Geometry: final body of the model. Coordinates: model frame, mm. A direction names the side the tool comes from. Coordinates: 2 decimals unless noted, no trailing zeros. Loops run counter-clockwise (first coordinate to the right, second up) from the corner with the lowest first, then second, coordinate; pieces in that order, holes last. Notation, with made-up numbers: (5, 35.25) -> (34, 35.25) arc R22 ccw to (34, 47.25) -> close; hole circle Ø6 at (33.5, -3.5). An arc over 180 degrees is marked (long way). One line per item, written item: value. Start each with the question number.
Item 1: Set-up query: faces 4 (the flat face through (-6, 0, -9)), 5 (the flat face through (-4.039, 1, -6)). Return all of +Z, -Z, +X, -X, +Y, -Y with unobstructed straight access to the full face (end or side cutting, diameter ignored); none if empty.
Item 2: Mould query, pull axis X, two halves, no side actions, for faces 1 (the flat face through (-8.661, 1, -6)), 2 (the flat face through (-6, 1, -12.7)), 3 (the flat face through (-11.541, 0.783, -1.127)). Classes: +X half, -X half, draft (parallel to the pull), parting line (faces both ways), or undercut.
Item 3: Section query B-B on y = 1.15. Return loops of the section in (x, z), then the cut area to 3 significant figures.
Item 4: Ray query, probe 1 along Z at (x, y) = (-7, 1.5); probe 2 along Z at (x, y) = (-8.5, 1.3). Return the intervals inside material, ascending. Write a range as from..to.
Item 5: Section query D-D on x = -1.25. Return loops of the section in (y, z).
Item 6: Section query C-C on z = -6.25. Return loops of the section in (x, y).
Item 7: Section query A-A on x = -7. Return loops of the section in (y, z).
Autodesk Inventor part; units mm, degrees
ref_plane "YZ Plane" through (0, 0, 0) normal (1, 0, 0) x (0, 1, 0)
ref_plane "XZ Plane" through (0, 0, 0) normal (0, 1, 0) x (-1, 0, 0)
ref_plane "XY Plane" through (0, 0, 0) normal (0, 0, 1) x (1, 0, 0)
sketch "Sketch1" plane through (0, 0, 0) normal (0, 1, 0) x (-1, 0, 0)
  line L0 (2.286, 0) -> (10.414, 0)
  line L1 (12.7, -2.286) -> (12.7, -10.414)
  line L2 (10.414, -12.7) -> (2.286, -12.7)
  line L3 (0, -10.414) -> (0, -2.286)
  line L4 (8.1534, -4.0386) -> (4.5466, -4.0386)
  line L5 (4.0386, -4.5466) -> (4.0386, -8.1534)
  line L6 (4.5466, -8.6614) -> (8.1534, -8.6614)
  line L7 (8.6614, -8.1534) -> (8.6614, -4.5466)
  line L8 (10.414, 0) -> (12.7, -2.286)
  line L9 (12.7, -10.414) -> (10.414, -12.7)
  line L10 (2.286, -12.7) -> (0, -10.414)
  line L11 (2.286, 0) -> (0, -2.286)
  arc A0 (8.6614, -4.5466) -> (8.1534, -4.0386) centre (8.1534, -4.5466) ccw
  arc A1 (8.1534, -8.6614) -> (8.6614, -8.1534) centre (8.1534, -8.1534) ccw
  arc A2 (4.0386, -8.1534) -> (4.5466, -8.6614) centre (4.5466, -8.1534) ccw
  arc A3 (4.5466, -4.0386) -> (4.0386, -4.5466) centre (4.5466, -4.5466) ccw
  line L12 (8.1534, -4.5466) -> (4.5466, -8.1534) construction
  line L13 (12.7, -10.414) -> (0, -2.286) construction
  point P0 (0, 0)
  point P1 (12.7, -12.7)
  point P2 (12.7, 0)
  point P3 (0, -12.7)
  point P4 (4.0386, -8.6614)
  point P5 (8.6614, -8.6614)
  point P6 (6.35, -6.35)
  dimension "d1" = 12.7
  dimension "d2" = 4.6228
  dimension "d3" = 2.286
  dimension "d4" = 2.286
  dimension "d5" = 2.286
  dimension "d6" = 2.286
  dimension "d7" = 2.286
  dimension "d8" = 2.286
  dimension "d9" = 2.286
  dimension "d10" = 2.286
  dimension "d11" = 0.508
extrude "Body" add sketch "Sketch1" along normal blind 1.5875
sketch "Sketch2" plane through (0, 1.5875, 0) normal (0, 1, 0) x (1, 0, 0)
  arc A0 (-8.1534, 8.6614) -> (-8.6614, 8.1534) centre (-8.1534, 8.1534) ccw construction
  arc A1 (-4.5466, 4.0386) -> (-4.0386, 4.5466) centre (-4.5466, 4.5466) ccw construction
  circle A2 centre (-6.35, 6.35) radius 2.1844
  line L0 (-8.1534, 8.1534) -> (-4.5466, 4.5466) construction
  point P0 (0, 0)
  dimension "d14" = 4.3688
surface extrude "Circle" sketch "Sketch2" against normal up to surface (1.5875 mm away) shown yes curves A2
pattern_of_one "Rectangular Pattern1"
equation "\"d22\" = d19"
Reply:
1. face 4: +Z, -Z, +X, -X, -Y
1. face 5: +Y, -Y
2. face 1: undercut
2. face 2: draft
2. face 3: -X half
3. outline: (-12.7, -10.41) -> (-10.41, -12.7) -> (-2.29, -12.7) -> (0, -10.41) -> (0, -2.29) -> (-2.29, 0) -> (-10.41, 0) -> (-12.7, -2.29) -> close; hole (-8.66, -8.15) arc R0.51 ccw to (-8.15, -8.66) -> (-4.55, -8.66) arc R0.51 ccw to (-4.04, -8.15) -> (-4.04, -4.55) arc R0.51 ccw to (-4.55, -4.04) -> (-8.15, -4.04) arc R0.51 ccw to (-8.66, -4.55) -> close
3. area: 130 mm²
4. probe 1: z = -12.7..-8.66, -4.04..0
4. probe 2: z = -12.7..-8.52, -4.18..0
5. outline: (0, -11.66) -> (1.59, -11.66) -> (1.59, -1.04) -> (0, -1.04) -> close
6. outline: (-12.7, 0) -> (-8.66, 0) -> (-8.66, 1.59) -> (-12.7, 1.59) -> close; (-4.04, 0) -> (0, 0) -> (0, 1.59) -> (-4.04, 1.59) -> close
7. outline: (0, -12.7) -> (1.59, -12.7) -> (1.59, -8.66) -> (0, -8.66) -> close; (0, -4.04) -> (1.59, -4.04) -> (1.59, 0) -> (0, 0) -> close
